Read the model definition and answer for the solid it produces. Units are mm, in the model's axes. A direction names the side the tool comes from. Give positions to 0.01 mm unless a question says otherwise; leave off trailing zeros. Write each loop counter-clockwise with the first axis right and the second up, starting at its lowest first coordinate (ties: lowest second). Pieces come first, ordered by that corner, then holes. Notation, with made-up numbers: (46, 36.25) - (65, 36.25) arc R31 ccw to (65, 67.25) - close; hole circle Ø2 at (47.5, -28.75). An arc over 180 degrees is marked (long way). Answer as CSV lines item,"result".
```python
from build123d import *

# Parameters (mm, degrees)
SKETCH_1_W                   = 25
SKETCH_1_H                   = 25
SKETCH_1_W_2                 = 21
SKETCH_1_H_2                 = 21
EXTRUDE_1_DEPTH              = 36
SKETCH_11_R                  = 2
CUT_EXTRUDE_3_DEPTH          = 7
CUT_EXTRUDE_START            = -19
SKETCH_11_3_R                = 2
CUT_EXTRUDE_11_DEPTH         = 32.457903246
CHAMFER_2_SIZE               = 1
CHAMFER_4_SIZE               = 1
CHAMFER_4_SIZE2              = 1.327044822
SKETCH_14_R                  = 7.5
CUT_EXTRUDE_6_DEPTH          = 5
CHAMFER_5_SIZE               = 0.5
CUT_EXTRUDE_8_DEPTH          = 50.497474683
HOLE_WIZARD_3_2_AT_2_COUNT   = 2
HOLE_WIZARD_3_2_AT_2_PITCH   = 13
HOLE_WIZARD_4_401_AT_2_COUNT = 2
HOLE_WIZARD_4_401_AT_2_PITCH = 16
CUT_EXTRUDE_13_DEPTH         = 3
CUT_EXTRUDE_14_DEPTH         = 3
SKETCH_25_R                  = 1.75
CUT_EXTRUDE_15_DEPTH         = 51.457903246
SKETCH_26_R                  = 6
CUT_EXTRUDE_16_DEPTH         = 5
CHAMFER_6_SIZE               = 1.5


with BuildPart() as part:
    # Sketch 1 → Extrude 1 (new body)
    with BuildSketch(Plane.XY):
        with Locations((12.5, 12.5)):
            Rectangle(SKETCH_1_W, SKETCH_1_H)
        with Locations((12.5, 12.5)):
            Rectangle(SKETCH_1_W_2, SKETCH_1_H_2, mode=Mode.SUBTRACT)
    extrude(amount=EXTRUDE_1_DEPTH)

    # Sketch 11 → Cut-Extrude 3 (cut)
    with BuildSketch(Plane(origin=(0, 25, 0), x_dir=(1, 0, 0), z_dir=(0, 1, 0))):
        with BuildLine():
            Line((25, -18.52949345), (25, -13.862588694))
            Line((25, -13.862588694), (15.357506109, -23.505082585))
            ThreePointArc((15.357506109, -23.505082585), (16.862903558, -24.03627397), (17.5, -25.5))
            ThreePointArc((17.5, -25.5), (17.47421651, -25.820108062), (17.397530829, -26.131962621))
            Line((17.397530829, -26.131962621), (25, -18.52949345))
        make_face()
        with BuildLine():
            Line((7.087167948, -15.115984981), (0, -22.203152929))
            Line((0, -22.203152929), (0, -26.870057685))
            Line((0, -26.870057685), (9.177993887, -17.692063798))
            ThreePointArc((9.177993887, -17.692063798), (7.447111922, -16.960372412), (7.087167948, -15.115984981))
        make_face()
        with Locations((9, -15.7)):
            Circle(SKETCH_11_R)
        with Locations((15.5, -25.5)):
            Circle(SKETCH_11_R)
    extrude(amount=-CUT_EXTRUDE_3_DEPTH, mode=Mode.SUBTRACT)

    # Sketch 11_3 → Cut-Extrude 11 (cut, through all)
    with BuildSketch(Plane(origin=(0, 25, 0), x_dir=(1, 0, 0), z_dir=(0, 1, 0)).offset(CUT_EXTRUDE_START)):
        with BuildLine():
            Line((25, -18.52949345), (25, -13.862588694))
            Line((25, -13.862588694), (15.357506109, -23.505082585))
            ThreePointArc((15.357506109, -23.505082585), (16.862903558, -24.03627397), (17.5, -25.5))
            ThreePointArc((17.5, -25.5), (17.47421651, -25.820108062), (17.397530829, -26.131962621))
            Line((17.397530829, -26.131962621), (25, -18.52949345))
        make_face()
        with Locations((15.5, -25.5)):
            Circle(SKETCH_11_3_R)
        with Locations((9, -15.7)):
            Circle(SKETCH_11_3_R)
        with BuildLine():
            Line((0, -22.203152929), (0, -26.870057685))
            Line((0, -26.870057685), (9.177993887, -17.692063798))
            ThreePointArc((9.177993887, -17.692063798), (7.447111922, -16.960372412), (7.087167948, -15.115984981))
            Line((7.087167948, -15.115984981), (0, -22.203152929))
        make_face()
    extrude(amount=-CUT_EXTRUDE_11_DEPTH, mode=Mode.SUBTRACT)

    # Hole Wizard M21: read off the stored shape, not the designer's step
    # Hole Wizard M21 outline → Hole Wizard M21 (revolve, cut)
    with BuildSketch(Plane(origin=(12, 0, 28.5), x_dir=(1, 0, 0), z_dir=(0, 0, 1))):
        Polygon((0, 23), (1.225, 23), (1.2, 23.025), (1.2, 25), (0, 25), align=None)
    revolve(axis=Axis((12, 0, 28.5), (0, 1, 0)), mode=Mode.SUBTRACT)

    # Chamfer 2
    chamfer_2_edges = [part.edges().sort_by_distance(p)[0] for p in [
        (0, 0, 31.435028843),
        (0, 0, 11.101576465),
    ]]
    chamfer(chamfer_2_edges, length=CHAMFER_2_SIZE)

    # Chamfer 4
    chamfer_4_edges = [part.edges().sort_by_distance(p)[0] for p in [
        (2, 12.5, 0),
    ]]
    chamfer_4_side = [part.faces().sort_by_distance(p)[0] for p in [
        (0.353553391, 13, 0),
    ]]
    chamfer(chamfer_4_edges, length=CHAMFER_4_SIZE, length2=CHAMFER_4_SIZE2, reference=chamfer_4_side[0])

    # Sketch 14 → Cut-Extrude 6 (cut)
    with BuildSketch(Plane.XZ):
        with Locations((30, 35.5)):
            Circle(SKETCH_14_R)
    extrude(amount=-CUT_EXTRUDE_6_DEPTH, mode=Mode.SUBTRACT)

    # Chamfer 5
    # the kernel refuses this chamfer: 0.5 mm, written as the material it takes off along each edge
    with BuildSketch(Plane(origin=(23, 5, 32.807417596), x_dir=(0, 0, -1), z_dir=(0, -1, 0))) as chamfer_5_piece_1:
        with BuildLine():
            Line((CHAMFER_5_SIZE, 0), (0.463529248, 0.196401008))
            ThreePointArc((0.463529248, 0.196401008), (0.235400494, 0.095152706), (0, 0))
            Line((0, 0), (CHAMFER_5_SIZE, 0))
        make_face()
    extrude(amount=3, mode=Mode.SUBTRACT)

    # Sketch 20 → Cut-Extrude 8 (cut, through all)
    with BuildSketch(Plane(origin=(2, 0, 0), x_dir=(0, 0, -1), z_dir=(1, 0, 0))):
        Polygon((-131.440037453, 23), (-36, 23), (-32, 23), (-32, 2), (-36, 2), (-131.440037453, 2), (-322.32011236, 2), (-322.32011236, 23), align=None)
    extrude(amount=-CUT_EXTRUDE_8_DEPTH, mode=Mode.SUBTRACT)

    # Sketch 15 → Hole Wizard 3.2 (revolve, cut)
    with BuildSketch(Plane(origin=(5, 0, 29.5), x_dir=(0, 0, -1), z_dir=(1, 0, 0))):
        Polygon((0, 0), (0, 2), (1.8, 2), (1.6, 1.8), (1.6, 0.2), (1.8, 0), align=None)
    hole_wizard_3_2 = revolve(axis=Axis((5, -6.35, 29.5), (0, 1, 0)), mode=Mode.SUBTRACT)

    # Hole Wizard 3.2 at 2: Hole Wizard 3.2 ×2
    with Locations(*[(i * HOLE_WIZARD_3_2_AT_2_PITCH, 0, 0) for i in range(1, HOLE_WIZARD_3_2_AT_2_COUNT)]):
        add(hole_wizard_3_2, mode=Mode.SUBTRACT)

    # Sketch 17 → Hole Wizard 4-401 (revolve, cut)
    with BuildSketch(Plane(origin=(0, 20, 13), x_dir=(0, 0, 1), z_dir=(0, 1, 0))):
        Polygon((0, 0), (0, 2), (1.651, 2), (1.4224, 1.839932557), (1.4224, 0.160067443), (1.651, 0), align=None)
    hole_wizard_4_401 = revolve(axis=Axis((-6.35, 20, 13), (1, 0, 0)), mode=Mode.SUBTRACT)

    # Hole Wizard 4-401 at 2: Hole Wizard 4-401 ×2
    with Locations(*[(0, -i * HOLE_WIZARD_4_401_AT_2_PITCH, 0) for i in range(1, HOLE_WIZARD_4_401_AT_2_COUNT)]):
        add(hole_wizard_4_401, mode=Mode.SUBTRACT)

    # Sketch 23 → Cut-Extrude 13 (cut)
    with BuildSketch(Plane.ZY):
        with BuildLine():
            Line((20, 25), (20, 19.5))
            ThreePointArc((20, 19.5), (20.878679656, 17.378679656), (23, 16.5))
            Line((23, 16.5), (24.5, 16.5))
            ThreePointArc((24.5, 16.5), (26.621320344, 17.378679656), (27.5, 19.5))
            Line((27.5, 19.5), (27.5, 25))
            Line((27.5, 25), (20, 25))
        make_face()
        with BuildLine():
            Line((20, 5.5), (20, 0))
            Line((20, 0), (27.5, 0))
            Line((27.5, 0), (27.5, 5.5))
            ThreePointArc((27.5, 5.5), (26.621320344, 7.621320344), (24.5, 8.5))
            Line((24.5, 8.5), (23, 8.5))
            ThreePointArc((23, 8.5), (20.878679656, 7.621320344), (20, 5.5))
        make_face()
    extrude(amount=-CUT_EXTRUDE_13_DEPTH, mode=Mode.SUBTRACT)

    # Sketch 24 → Cut-Extrude 14 (cut)
    with BuildSketch(Plane(origin=(25, 0, 0), x_dir=(0, 0, -1), z_dir=(1, 0, 0))):
        with BuildLine():
            Line((-13.5, 25), (-13.5, 19.5))
            ThreePointArc((-13.5, 19.5), (-14.378679656, 17.378679656), (-16.5, 16.5))
            Line((-16.5, 16.5), (-18, 16.5))
            ThreePointArc((-18, 16.5), (-20.121320344, 17.378679656), (-21, 19.5))
            Line((-21, 19.5), (-21, 25))
            Line((-21, 25), (-13.5, 25))
        make_face()
        with BuildLine():
            Line((-13.5, 0), (-13.5, 5.5))
            ThreePointArc((-13.5, 5.5), (-14.378679656, 7.621320344), (-16.5, 8.5))
            Line((-16.5, 8.5), (-18, 8.5))
            ThreePointArc((-18, 8.5), (-20.121320344, 7.621320344), (-21, 5.5))
            Line((-21, 5.5), (-21, 0))
            Line((-21, 0), (-13.5, 0))
        make_face()
    extrude(amount=-CUT_EXTRUDE_14_DEPTH, mode=Mode.SUBTRACT)

    # Sketch 25 → Cut-Extrude 15 (cut, through all)
    with BuildSketch(Plane.XZ):
        with Locations(Location((10, 6, 0), (0, 0, 270))):
            Circle(SKETCH_25_R)
    extrude(amount=-CUT_EXTRUDE_15_DEPTH, mode=Mode.SUBTRACT)

    # Sketch 26 → Cut-Extrude 16 (cut)
    with BuildSketch(Plane.XZ.offset(-5)):
        with Locations((30, 35.5)):
            Circle(SKETCH_26_R)
    extrude(amount=-CUT_EXTRUDE_16_DEPTH, mode=Mode.SUBTRACT)

    # Sketch 27 → Hole Wizard M31 (revolve, cut)
    with BuildSketch(Plane(origin=(18, 25, 29.5), x_dir=(0, 0, 1), z_dir=(1, 0, 0))):
        Polygon((0, 0), (0, 2), (1.8, 2), (1.575, 1.775), (1.575, 0.225), (1.8, 0), align=None)
    revolve(axis=Axis((18, 31.35, 29.5), (0, -1, 0)), mode=Mode.SUBTRACT)

    # Chamfer 6
    chamfer_6_edges = [part.edges().sort_by_distance(p)[0] for p in [
        (10, 2, 7.75),
        (10, 23, 7.75),
    ]]
    chamfer(chamfer_6_edges, length=CHAMFER_6_SIZE)

    # Sketch 29 → Hole Wizard M32 (revolve, cut)
    with BuildSketch(Plane(origin=(25, 18, 29.5), x_dir=(0, 0, -1), z_dir=(0, 1, 0))):
        Polygon((0, 0), (0, 2), (1.8, 2), (1.7, 1.9), (1.7, 0.1), (1.8, 0), align=None)
    revolve(axis=Axis((31.35, 18, 29.5), (-1, 0, 0)), mode=Mode.SUBTRACT)


solid = part.part
```
(1) A cutting plane is placed at A-A (y = 12.25). Write down the section's boundary in (x, z).
Worked out:
outline,"(0, 0) - (1, 0) - (2, 1.33) - (2, 32) - (0, 32) - close; (23, 0) - (25, 0) - (25, 36) - (23, 36) - close"
(2) Find the intervals of material crossed by L1, parallel to X at y = 1.1, z = 29.5; L2, parallel to X at y = 6.75, z = 4, in increasing order.
Worked out:
L1,"x = 0 to 3.4, 6.6 to 16.4, 19.6 to 25"
L2,"x = 0 to 2, 23 to 25"
(3) The mould has two halves that part along Z. Classify faces 1 (the flat face through (13, 0, 18)), 2 (the cylindrical face through (16.414, 0.989, 29.708)), 3 (the flat face through (11, 1, 36)): +Z half, -Z half, draft (parallel to the pull), parting line (faces both ways), or undercut.
Worked out:
face 1,"draft"
face 2,"undercut"
face 3,"+Z half"
(4) A cutting plane is placed at C-C (x = 18). Count the separate pieces of the cut face and the enclosed holes in it, and give its area (3 significant figures).
Worked out:
separate pieces,"6"
enclosed holes,"0"
area,"112 mm^2"
(5) For faces 4 (the cylindrical face through (0.99, 17.4, 20.86)), 5 (the cylindrical face through (24.18, 7.46, 34.04)), 6 (the flat face through (1, 3, 27.5)), 7 (the cylindrical face through (0.99, 2.8, 13.76)), 8 (the flat face through (6.05, 1.01, 20.82)), determine the directions among +Z, -Z, +X, -X, +Y, -Y from which every point of the face is accessible in a straight line to the end or side of a thin tool.
Worked out:
face 4,"-X, +Y"
face 5,"+X, -Y"
face 6,"-X, -Y"
face 7,"-X"
face 8,"+Y, -Y"
(6) A cutting plane is placed at B-B (z = 15.7). Write down the section's boundary in (x, y).
Worked out:
outline,"(0, 1) - (1, 0) - (6.5, 0) - (6.5, 2) - (2, 2) - (2, 23) - (6.5, 23) - (6.5, 25) - (0, 25) - close; (11, 0) - (22, 0) - (22, 2) - (11, 2) - close; (11, 23) - (22, 23) - (22, 25) - (11, 25) - close; (23, 8.39) - (25, 8.39) - (25, 16.61) - (23, 16.61) - close"
(7) Each of these flat-tipped pins is pushed along its axis until it touches: P1, Ø1.2, axis at x = 24, z = 17, coming from the -Y side; P2, Ø1, axis at y = 1, z = 15, coming from the +X side; P3, Ø1.2, axis at x = 1.5, z = 24, coming from the +Y side. Where does it stop, or does it pass through?
Worked out:
P1,"stops at y = 8.5"
P2,"stops at x = 22"
P3,"stops at y = 16.5"
(8) A cutting plane is placed at D-D (y = 4). Write down the section's boundary in (x, z), and give its area (4 significant figures).
Worked out:
outline,"(0, 0) - (1, 0) - (2, 1.33) - (2, 11.35) - (1.84, 11.58) - (0.16, 11.58) - (0, 11.35) - close; (0, 14.65) - (0.16, 14.42) - (1.84, 14.42) - (2, 14.65) - (2, 20) - (0, 20) - close; (0, 27.5) - (2, 27.5) - (2, 32) - (0, 32) - close; (23, 0) - (25, 0) - (25, 13.5) - (23, 13.5) - close; (23, 21) - (25, 21) - (25, 29.91) arc R7.5 cw to (23.2, 32.34) - (23, 32.31) - close"
area,"89.75 mm^2"
